Study the drawing (mm; zero at the part's minimum x, y, z) and answer. A direction names the side the tool comes from. Give positions to 0.01 mm unless a question says otherwise; leave off trailing zeros. Write each loop counter-clockwise with the first axis right and the second up, starting at its lowest first coordinate (ties: lowest second). Pieces come first, ordered by that corner, then holes.
1) Find section C-C (z = 9.75). Determine the outline of the cut face in (x, y), plus the area to 3 significant figures.
2) Given pin 1 Ø3.5 at (x, z) = (70.5, 4.5) entering from +Y; pin 2 Ø10 at (x, y) = (18.5, 34) entering from +Z; pin 3 Ø7.5 at (y, z) = (44.5, 2) entering from -X, each flat-ended and moving along its own axis, determine where each tip first touches the part or whether it passes through.
3) Determine the mould class of the marked faces 1, 2, 3 and 4 for opening direction Y: pulls with the +Y half, pulls with the -Y half, needs draft (parallel to the pull), parting line crosses it, or undercut.
4) Find section B-B (y = 14.5). Determine the outline of the cut face in (x, z).
5) Find section D-D (x = 25.5). Determine the outline of the cut face in (y, z), plus the area to 3 significant figures.
6) A tool of negligible diameter and unlimited length cuts with its end or side. For the marked faces 5, 6, 7, 8 and 9, from which of +Z, -Z, +X, -X, +Y, -Y can it reach the whole face along a straight path? Write none if from no direction.
7) Find section A-A (z = 15). Determine the outline of the cut face in (x, y), plus the area to 3 significant figures.
8) Straight lines are drawn through the part: probe 1 along X at (y, z) = (3, 14.75); probe 2 along Z at (x, y) = (75, 1); probe 3 along Y at (x, z) = (40, 4). For each, find the intervals that lie inside material, in ascending order.
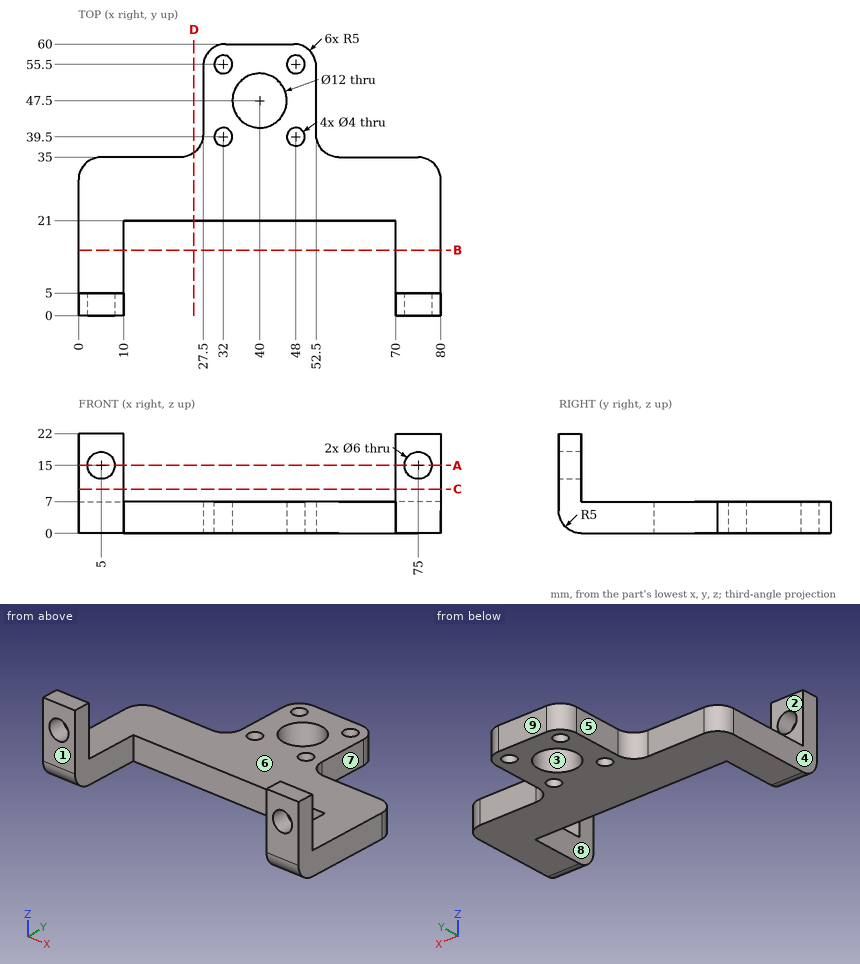
Results:
1. outline: (0, 0) - (10, 0) - (10, 5) - (0, 5) - close; (70, 0) - (80, 0) - (80, 5) - (70, 5) - close
1. area: 100 mm2
2. pin 1: stops at y = 35
2. pin 2: stops at z = 7
2. pin 3: stops at x = 27.5
3. face 1: pulls with the -Y half
3. face 2: pulls with the +Y half
3. face 3: undercut
3. face 4: needs draft
4. outline: (0, 0) - (10, 0) - (10, 7) - (0, 7) - close; (70, 0) - (80, 0) - (80, 7) - (70, 7) - close
5. outline: (21, 0) - (36, 0) - (36, 7) - (21, 7) - close
5. area: 105 mm2
6. face 5: +Z, -Z, -X, +Y
6. face 6: +Z, +X, -X, +Y
6. face 7: +Z, -Z, +X, +Y
6. face 8: +Z, -Z, -Y
6. face 9: +Z, -Z, +X, -X, +Y
7. outline: (0, 0) - (2, 0) - (2, 5) - (0, 5) - close; (8, 0) - (10, 0) - (10, 5) - (8, 5) - close; (70, 0) - (72, 0) - (72, 5) - (70, 5) - close; (78, 0) - (80, 0) - (80, 5) - (78, 5) - close
7. area: 40.0 mm2
8. probe 1: x = 0 to 2.01, 7.99 to 10, 70 to 72.01, 77.99 to 80
8. probe 2: z = 2 to 12, 18 to 22
8. probe 3: y = 21 to 41.5, 53.5 to 60
